Check sheet for the modelled part. Datum: model origin and axes. Units: mm. A direction names the side the tool comes from. Coordinates: 2 decimals unless noted, no trailing zeros. Write each loop counter-clockwise with the first axis right and the second up, starting at its lowest first coordinate (ties: lowest second). Pieces come first, ordered by that corner, then holes. Notation, with made-up numbers: (24, 20.25) - (44, 20.25) arc R35 ccw to (44, 55.25) - close; hole circle Ø2 at (-18.5, 80). An arc over 180 degrees is marked (long way). Use one line per item in the form item = value. Start each with the question number.
1. Cross-section at A-A on y = 0. Record the boundary of the cut face in (x, z).
2. Cross-section at D-D on y = -5. Record the boundary of the cut face in (x, z).
3. Cross-section at B-B on x = 12. Record the boundary of the cut face in (y, z), then the cut area to 3 significant figures.
4. Scan lines: line 1 along Y through (x, z) = (12, -2.95); line 2 along Y through (x, z) = (12, -1.95); line 3 along Z through (x, y) = (2.25, -0.5). Record each from-to range of solid material in increasing order.
5. Draft check along X on faces 1 (the face through (11.41, 6.79, -2.99)), 2 (the face through (14, 0, -2)), 3 (the face through (13, 6, -2)), 4 (the face through (12, 0, -4)). Enter one of: +X half, -X half, draft (parallel to the pull), parting line (faces both ways), or undercut.
6. Go/stop test with flat-tipped pins: pin 1 Ø1.8 at (x, y) = (12, 6.25) entering from -Z; pin 2 Ø1.5 at (x, y) = (3.5, -6.5) entering from -Z; pin 3 Ø1 at (x, z) = (9, -1.5) entering from -Y. Record where each tip stops, or that it passes through.
7. Tool access check on faces 5 (the face through (6.9, 8.51, -1.54)), 6 (the face through (0, -2, -4)), 7 (the face through (12.577, 5.141, -0.986)). Record the directions out of +Z, -Z, +X, -X, +Y, -Y that give a thin tool (end or side, any length) a straight path to the whole face; none if there is none.
8. Cross-section at C-C on z = -1.1. Record the boundary of the cut face in (x, y).
```python
from build123d import *

# Parameters (mm, degrees)
SKETCH1_R           = 10
BOSS_EXTRUDE1_DEPTH = 4
BODY_START          = -3
SKETCH2_R           = 10
BODY_HOLE_DEPTH     = 2
BOSS_EXTRUDE2_START = -3
SKETCH11_R          = 2
BOSS_EXTRUDE2_DEPTH = 2
SKETCH4_R           = 0.75
CUT_EXTRUDE2_DEPTH  = 6
SKETCH3_R           = 0.8
SCREW_HOLES_DEPTH   = 6
SKETCH6_R           = 1.25
SCREW_HEADS_DEPTH   = 2
CUT_REVOLVE1_ANGLE  = 180
CUT_EXTRUDE1_DEPTH  = 15.000000004


with BuildPart() as part:
    # Sketch1 → Boss-Extrude1 (new body)
    with BuildSketch(Plane.XY):
        with Locations((4e-09, 0)):
            Circle(SKETCH1_R)
        with BuildLine():
            Line((14.000000004, 10), (4e-09, 10))
            ThreePointArc((4e-09, 10), (7.071067816, 7.071067812), (10.000000004, 0))
            ThreePointArc((10.000000004, 0), (7.071067816, -7.071067812), (4e-09, -10))
            Line((4e-09, -10), (14.000000004, -10))
            Line((14.000000004, -10), (14.000000004, 10))
        make_face()
    extrude(amount=-BOSS_EXTRUDE1_DEPTH)

    # Sketch2 → Body Hole (cut)
    with BuildSketch(Plane.XY.offset(BODY_START)):
        with Locations((4e-09, 0)):
            Circle(SKETCH2_R)
        with BuildLine():
            Line((10.000000004, 10), (4e-09, 10))
            ThreePointArc((4e-09, 10), (7.071067816, 7.071067812), (10.000000004, 0))
            Line((10.000000004, 0), (10.000000004, 10))
        make_face()
        with BuildLine():
            Line((10.000000004, -10), (10.000000004, 0))
            ThreePointArc((10.000000004, 0), (7.071067814, -7.071067813), (0, -10))
            Line((0, -10), (10.000000004, -10))
        make_face()
    extrude(amount=-BODY_HOLE_DEPTH, mode=Mode.SUBTRACT)

    # Sketch11 → Boss-Extrude2 (add)
    with BuildSketch(Plane.XY.offset(BOSS_EXTRUDE2_START)):
        with Locations((4e-09, 0)):
            Circle(SKETCH11_R)
    extrude(amount=-BOSS_EXTRUDE2_DEPTH)

    # Sketch4 → Cut-Extrude2 (cut, through all)
    with BuildSketch(Plane.XY):
        with Locations((4e-09, 0)):
            Circle(SKETCH4_R)
    extrude(amount=-CUT_EXTRUDE2_DEPTH, mode=Mode.SUBTRACT)

    # Sketch3 → Screw Holes (cut, through all)
    with BuildSketch(Plane.XY):
        with Locations((12.000000004, 6.25)):
            Circle(SKETCH3_R)
        with Locations((12.000000004, -6.25)):
            Circle(SKETCH3_R)
    extrude(amount=-SCREW_HOLES_DEPTH, mode=Mode.SUBTRACT)

    # Sketch6 → Screw Heads (cut)
    with BuildSketch(Plane.XY):
        with Locations((12.000000004, 6.25)):
            Circle(SKETCH6_R)
    extrude(amount=-SCREW_HEADS_DEPTH, mode=Mode.SUBTRACT)

    # Sketch9 → Cut-Revolve1 (revolve, cut)
    with BuildSketch(Plane(origin=(0, 0, 0), x_dir=(0, 0, -1), z_dir=(1, 0, 0))):
        with BuildLine():
            Line((-2, 12), (-2, 2.75))
            Line((-2, 2.75), (-1.680646386, 2.75))
            ThreePointArc((-1.680646386, 2.75), (2.550167787, 9.407443861), (10, 12))
            Line((10, 12), (-2, 12))
        make_face()
    revolve(axis=Axis((0, 0, 0), (0, 0, 1)), revolution_arc=CUT_REVOLVE1_ANGLE, mode=Mode.SUBTRACT)

    # Sketch10 → Cut-Extrude1 (cut, through all)
    with BuildSketch(Plane(origin=(0, 0, 0), x_dir=(0, 0, -1), z_dir=(1, 0, 0))):
        with BuildLine():
            ThreePointArc((10, 12), (1.514718626, 8.485281374), (-2, 0))
            Line((-2, 0), (-2, 12))
            Line((-2, 12), (10, 12))
        make_face()
        with BuildLine():
            ThreePointArc((-2, 0), (1.514718626, -8.485281374), (10, -12))
            Line((10, -12), (-2, -12))
            Line((-2, -12), (-2, 0))
        make_face()
    extrude(amount=CUT_EXTRUDE1_DEPTH, mode=Mode.SUBTRACT)


solid = part.part
```
Final values:
q1.outline = (-9.75, -3) - (-2, -3) - (-2, -5) - (-0.75, -5) - (-0.75, 0) - (-6.63, 0) arc R12 ccw to start; (0.75, -5) - (2, -5) - (2, -3) - (10, -3) - (10, -4) - (14, -4) - (14, 0) - (0.75, 0) - close
q2.outline = (-8.37, -3) - (10, -3) - (10, -4) - (14, -4) - (14, 0) - (-4.36, 0) arc R10.91 ccw to start
q3.outline = (-10, -4) - (-7.05, -4) - (-7.05, -0.29) arc R12 ccw to (-10, -3.37) - close; (-5.45, -4) - (5.45, -4) - (5.45, -2) - (5, -2) - (5, 0) - (-5.45, 0) - close; (7.05, -4) - (10, -4) - (10, -3.37) arc R12 ccw to (7.5, -0.63) - (7.5, -2) - (7.05, -2) - close
q3.area = 55.9 mm²
q4.line_1 = -9.71 to -7.05, -5.45 to 5.45, 7.05 to 9.71
q4.line_2 = -8.9 to -7.05, -5.45 to 5, 7.5 to 8.9
q4.line_3 = -3 to 0
q5.face_1 = undercut
q5.face_2 = +X half
q5.face_3 = undercut
q5.face_4 = draft
q6.pin_1 = -4
q6.pin_2 = -3
q6.pin_3 = -8.94
q7.face_5 = +Z, +X, -X, +Y
q7.face_6 = -Z
q7.face_7 = +Z
q8.outline = (0, -8.05) - (14, -8.05) - (14, 8.05) - (0, 8.05) arc R8.05 ccw to start; hole circle Ø1.5 at (0, 0); hole circle Ø2.5 at (12, 6.25); hole circle Ø1.6 at (12, -6.25)
